Check sheet for the modelled part. Datum: model origin and axes. Units: mm. A direction names the side the tool comes from. Coordinates: 2 decimals unless noted, no trailing zeros. Write each loop counter-clockwise with the first axis right and the second up, starting at its lowest first coordinate (ties: lowest second). Pieces come first, ordered by that corner, then holes. Notation, with made-up numbers: (35.5, 22.25) -> (90.5, 22.25) arc R20 cw to (90.5, 59.25) -> close; hole circle Ø7 at (66, 26.5). An arc over 180 degrees is marked (long way). One line per item, written item: value. Start each with the question number.
1) Sectioned sample at A-A on z = 249.75. Enter the section's corners in (x, y).
2) Scan lines: line 1 along Z through (x, y) = (0.5, 25); line 2 along X through (y, z) = (69, 362); line 3 along Y through (x, z) = (1, 348.3). Record each from-to range of solid material in increasing order. Write a range as [from, to].
3) Sectioned sample at C-C on y = 104.5. Enter the section's corners in (x, z).
4) Draft check along Y on faces 1 (the cylindrical face through (1.014, 14.599, 279.117)), 2 (the cylindrical face through (1.014, 14.599, 253.567)), 3 (the flat face through (8, 2, 192)), 4 (the flat face through (8, 0, 192)). Enter one of: +Y half, -Y half, draft (parallel to the pull), parting line (faces both ways), or undercut.
5) Set-up check for faces 5 (the flat face through (1.6, 10.1, 380)), 6 (the flat face through (1.6, 10.1, 10)), 7 (the cylindrical face through (1.014, 14.199, 352.117)), 8 (the flat face through (2, 60, 192)): record each of +Z, -Z, +X, -X, +Y, -Y from which the full face is reachable in a straight line by a thin tool's end or side.
6) Gauge pin test, flat ends, axial feed: P1, Ø2, axis at y = 46.5, z = 47.5, coming from the +X side; P2, Ø2, axis at x = 0.5, z = 385, coming from the -Y side; P3, Ø4.5, axis at y = 68.6, z = 314.8, coming from the -X side; P4, Ø2.5, axis at x = 6, z = 155, coming from the +Y side. Record the tip position at first contact, or that the pin passes through.
7) Sectioned sample at B-B on z = 327. Enter the section's corners in (x, y), plus the area to 3 significant figures.
```python
from build123d import *

# Parameters (mm, degrees)
FLANGE_BASE1_DEPTH    = 390
ESBO_O6_R             = 2
ESBO_O6_R_2           = 3.85
ESBO_O6_W             = 10
ESBO_O6_H             = 26
CORTE_EXTRUS_O1_DEPTH = 98
ESBO_O7_R             = 2.25
CORTE_EXTRUS_O2_DEPTH = 98
ESBO_O8_W             = 3
ESBO_O8_H             = 94
CORTE_EXTRUS_O3_DEPTH = 10
ESBO_O9_W             = 384
ESBO_O9_H             = 2.5
CORTE_EXTRUS_O4_DEPTH = 10


# Sheet-metal steps are written as plain solids
with BuildPart() as part:
    # Esboço1 → Flange-base1 (new body)
    with BuildSketch(Plane.XY):
        with BuildLine():
            Line((0, 120), (0, 3.8))
            ThreePointArc((0, 3.8), (1.112994231, 1.112994231), (3.8, 0))
            Line((3.8, 0), (12, 0))
            Line((12, 0), (12, 2))
            Line((12, 2), (3.8, 2))
            ThreePointArc((3.8, 2), (2.527207794, 2.527207794), (2, 3.8))
            Line((2, 3.8), (2, 120))
            Line((2, 120), (0, 120))
        make_face()
    extrude(amount=FLANGE_BASE1_DEPTH)

    # Esboço6 → Corte-extrusão1 (cut)
    with BuildSketch(Plane(origin=(12, 0, 0), x_dir=(0, 0, -1), z_dir=(1, 0, 0))):
        with Locations(Location((-314.8, 25, 0), (0, 0, 90))):
            Circle(ESBO_O6_R)
        with Locations(Location((-314.8, 68.6, 0), (0, 0, 90))):
            Circle(ESBO_O6_R)
        with Locations(Location((-238, 25, 0), (0, 0, 90))):
            Circle(ESBO_O6_R)
        with Locations(Location((-238, 68.6, 0), (0, 0, 90))):
            Circle(ESBO_O6_R)
        with Locations(Location((-275.3, 15.1, 0), (0, 0, 90))):
            Circle(ESBO_O6_R_2)
        with Locations(Location((-249.75, 15.1, 0), (0, 0, 90))):
            Circle(ESBO_O6_R_2)
        with Locations(Location((-229.2, 18.4, 0), (0, 0, 90))):
            Circle(ESBO_O6_R_2)
        with Locations(Location((-190, 114.2, 0), (0, 0, 90))):
            Circle(ESBO_O6_R)
        with Locations(Location((-113, 114.2, 0), (0, 0, 90))):
            Circle(ESBO_O6_R)
        with Locations(Location((-348.3, 14.7, 0), (0, 0, 90))):
            Circle(ESBO_O6_R_2)
        with Locations((-5, 13)):
            Rectangle(ESBO_O6_W, ESBO_O6_H)
        with Locations((-385, 13)):
            Rectangle(ESBO_O6_W, ESBO_O6_H)
    extrude(amount=-CORTE_EXTRUS_O1_DEPTH, mode=Mode.SUBTRACT)

    # Esboço7 → Corte-extrusão2 (cut)
    with BuildSketch(Plane(origin=(0, 2, 0), x_dir=(1, 0, 0), z_dir=(0, 1, 0))):
        with Locations(Location((8, -350, 0), (0, 0, 270))):
            Circle(ESBO_O7_R)
        with Locations(Location((8, -288, 0), (0, 0, 270))):
            Circle(ESBO_O7_R)
        with Locations(Location((8, -226, 0), (0, 0, 270))):
            Circle(ESBO_O7_R)
        with Locations(Location((8, -164, 0), (0, 0, 270))):
            Circle(ESBO_O7_R)
        with Locations(Location((8, -102, 0), (0, 0, 270))):
            Circle(ESBO_O7_R)
        with Locations(Location((8, -40, 0), (0, 0, 270))):
            Circle(ESBO_O7_R)
    extrude(amount=-CORTE_EXTRUS_O2_DEPTH, mode=Mode.SUBTRACT)

    # Esboço8 → Corte-extrusão3 (cut)
    with BuildSketch(Plane.ZY):
        with Locations((1.5, 73)):
            Rectangle(ESBO_O8_W, ESBO_O8_H)
        with Locations((388.5, 73)):
            Rectangle(ESBO_O8_W, ESBO_O8_H)
    extrude(amount=-CORTE_EXTRUS_O3_DEPTH, mode=Mode.SUBTRACT)

    # Esboço9 → Corte-extrusão4 (cut)
    with BuildSketch(Plane(origin=(2, 0, 0), x_dir=(0, 0, -1), z_dir=(1, 0, 0))):
        with Locations((-195, 118.75)):
            Rectangle(ESBO_O9_W, ESBO_O9_H)
    extrude(amount=-CORTE_EXTRUS_O4_DEPTH, mode=Mode.SUBTRACT)


solid = part.part
```
Answers:
1. outline: (0, 3.8) arc R3.8 ccw to (3.8, 0) -> (12, 0) -> (12, 2) -> (3.8, 2) arc R1.8 cw to (2, 3.8) -> (2, 11.25) -> (0, 11.25) -> close; (0, 18.95) -> (2, 18.95) -> (2, 117.5) -> (0, 117.5) -> close
2. line 1: z = [10, 236], [240, 312.8], [316.8, 380]
2. line 2: x = [0, 2]
2. line 3: y = [1.23, 10.85], [18.55, 117.5]
3. outline: (0, 3) -> (2, 3) -> (2, 387) -> (0, 387) -> close
4. face 1: undercut
4. face 2: undercut
4. face 3: +Y half
4. face 4: -Y half
5. face 5: +Z, +X, -X, -Y
5. face 6: -Z, +X, -X, -Y
5. face 7: +X, -X
5. face 8: +Z, -Z, +X, +Y
6. P1: stops at x = 2
6. P2: stops at y = 26
6. P3: stops at x = 0
6. P4: stops at y = 2
7. outline: (0, 3.8) arc R3.8 ccw to (3.8, 0) -> (12, 0) -> (12, 2) -> (3.8, 2) arc R1.8 cw to (2, 3.8) -> (2, 117.5) -> (0, 117.5) -> close
7. area: 253 mm2
